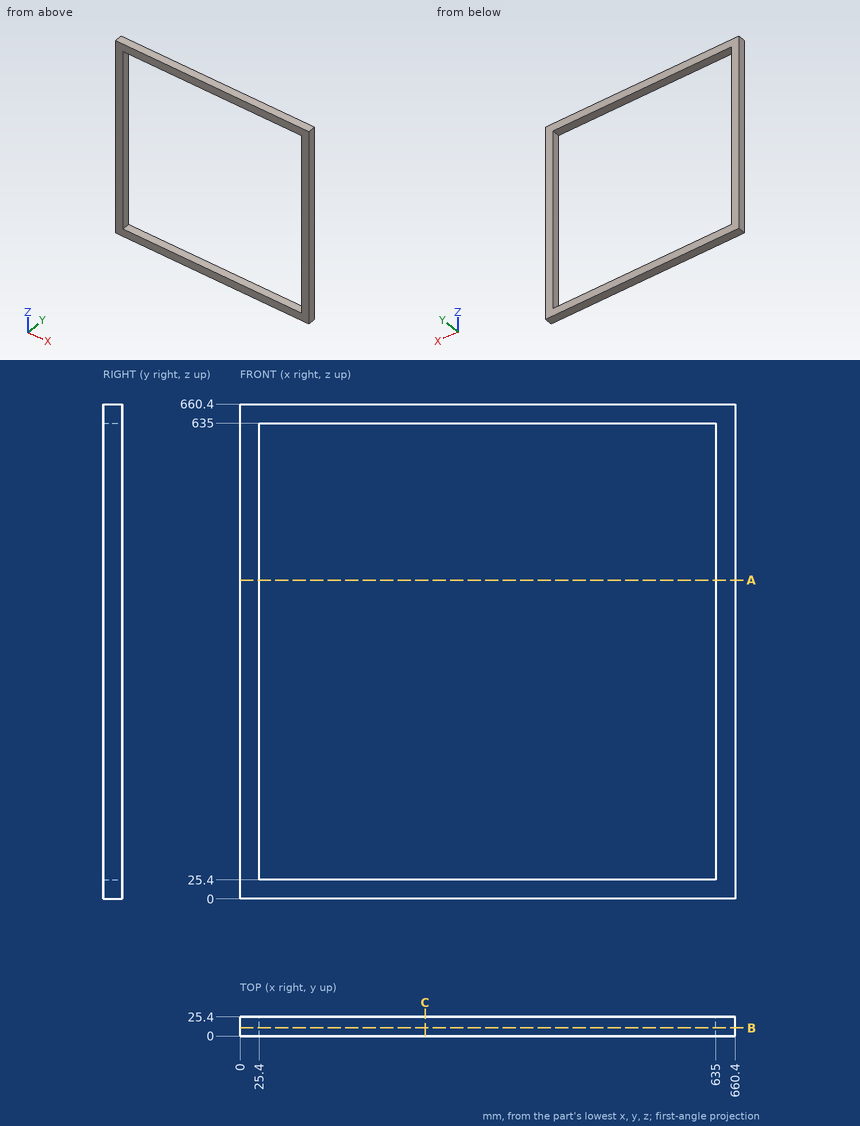
Could you check a few things on this drawing? It's one solid part, dimensions in mm from its lowest x, y, z. Coordinates: 2 decimals unless noted, no trailing zeros. Order: outer loops, then holes, each group sorted by start corner. A loop starts at its lowest first (then second) coordinate and runs counter-clockwise, first axis right, second up.
1) Imagine slicing it at C-C on x = 247. List the corners of the cut face in (y, z) for me, and give its area (3 significant figures).
2) Imagine slicing it at B-B on y = 10.75. List the corners of the cut face in (x, z) for me.
3) Imagine slicing it at A-A on z = 425.5. List the corners of the cut face in (x, y) for me.
4) I need wall thicknesses on line 1 (X direction, y = 4.25, z = 490.5). Which ranges of the line are inside material? Lowest first, please.
Response values:
1. outline: (0, 0) - (25.4, 0) - (25.4, 25.4) - (0, 25.4) - close; (0, 635) - (25.4, 635) - (25.4, 660.4) - (0, 660.4) - close
1. area: 1,290 mm2
2. outline: (0, 0) - (660.4, 0) - (660.4, 660.4) - (0, 660.4) - close; hole (25.4, 25.4) - (635, 25.4) - (635, 635) - (25.4, 635) - close
3. outline: (0, 0) - (25.4, 0) - (25.4, 25.4) - (0, 25.4) - close; (635, 0) - (660.4, 0) - (660.4, 25.4) - (635, 25.4) - close
4. line 1: x = 0 to 25.4, 635 to 660.4
